Here's how the part is built. I have some questions about the finished solid (model axes, mm). Face numbers are marked on the shaded views. Give positions to 0.01 mm unless a question says otherwise; leave off trailing zeros. Loops run counter-clockwise (first coordinate to the right, second up) from the corner with the lowest first, then second, coordinate; pieces in that order, holes last. Notation, with made-up numbers: (75, -10.75) - (122, -10.75) arc R26 cw to (122, 13.25) - close; hole circle Ø9 at (-3, 63). An arc over 180 degrees is marked (long way). Use one line per item in the form item = value.
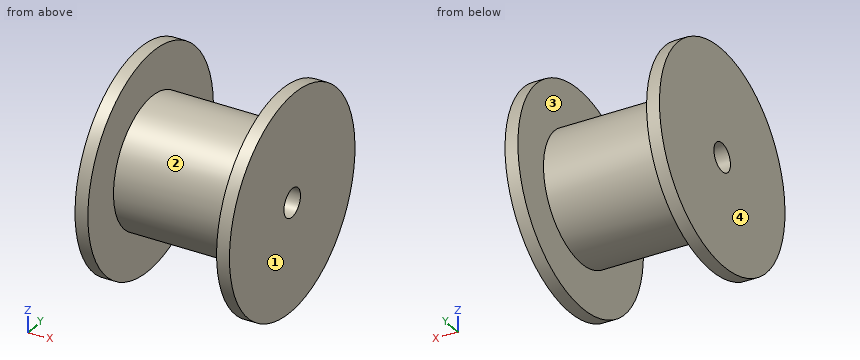
from build123d import *

# Parameters (mm, degrees)
CROQUIS1_R              = 76
SALIENTE_EXTRUIR1_DEPTH = 9
CROQUIS2_R              = 45
SALIENTE_EXTRUIR2_DEPTH = 90
CROQUIS3_R              = 76
SALIENTE_EXTRUIR3_DEPTH = 9
CROQUIS4_R              = 10
CORTAR_EXTRUIR1_DEPTH   = 108


with BuildPart() as part:
    # Croquis1 → Saliente-Extruir1 (new body)
    with BuildSketch(Plane(origin=(0, 0, 0), x_dir=(0, 0, -1), z_dir=(1, 0, 0))):
        Circle(CROQUIS1_R)
    extrude(amount=SALIENTE_EXTRUIR1_DEPTH)

    # Croquis2 → Saliente-Extruir2 (add)
    with BuildSketch(Plane(origin=(9, 0, 0), x_dir=(0, 0, -1), z_dir=(1, 0, 0))):
        with Locations(Location((0, 0, 0), (0, 0, 180))):
            Circle(CROQUIS2_R)
    extrude(amount=SALIENTE_EXTRUIR2_DEPTH)

    # Croquis3 → Saliente-Extruir3 (add)
    with BuildSketch(Plane(origin=(99, 0, 0), x_dir=(0, 0, -1), z_dir=(1, 0, 0))):
        Circle(CROQUIS3_R)
    extrude(amount=SALIENTE_EXTRUIR3_DEPTH)

    # Croquis4 → Cortar-Extruir1 (cut)
    with BuildSketch(Plane(origin=(108, 0, 0), x_dir=(0, 0, -1), z_dir=(1, 0, 0))):
        Circle(CROQUIS4_R)
    extrude(amount=-CORTAR_EXTRUIR1_DEPTH, mode=Mode.SUBTRACT)


solid = part.part
(1) If I drill on probe 1 along X at (y, z) = (12.5, 46.5); probe 2 along Y at (x, z) = (70.5, 0); probe 3 along Y at (x, z) = (22, -5), over which ranges is the centre line in solid material (lowest first)?
Geometry says:
probe_1 = 0 to 9, 99 to 108
probe_2 = -45 to -10, 10 to 45
probe_3 = -44.72 to -8.66, 8.66 to 44.72
(2) If we section it at C-C (x = 16.5): List the corners of the cut face in (y, z) for me, plus the area to 3 significant figures.
Geometry says:
outline = circle Ø90 at (0, 0); hole circle Ø20 at (0, 0)
area = 6,050 mm²
(3) For P1, Ø4, axis at x = 38, y = -29, coming from the +Z side; P2, Ø8, axis at x = 68.5, z = 18, coming from the -Y side; P3, Ø1.5, axis at x = 22.5, z = 21, coming from the +Y side, each with a flat end and sliding along its axis, tell me the tip position at first contact or that it passes through.
Geometry says:
P1 = 36
P2 = -42.77
P3 = 40.19
(4) If we section it at A-A (z = 0): List the corners of the cut face in (x, y) for me.
Geometry says:
outline = (0, -76) - (9, -76) - (9, -45) - (99, -45) - (99, -76) - (108, -76) - (108, -10) - (0, -10) - close; (0, 10) - (108, 10) - (108, 76) - (99, 76) - (99, 45) - (9, 45) - (9, 76) - (0, 76) - close
(5) If we section it at D-D (z = 59): List the corners of the cut face in (x, y) for me.
Geometry says:
outline = (0, -47.91) - (9, -47.91) - (9, 47.91) - (0, 47.91) - close; (99, -47.91) - (108, -47.91) - (108, 47.91) - (99, 47.91) - close
(6) Thinking about a two-plate mould opening in X: for the marked faces 1, 2, 3 and 4, which applies, pulls with the +X half, pulls with the -X half, needs draft (parallel to the pull), parting line crosses it, or undercut?
Geometry says:
face_1 = pulls with the +X half
face_2 = undercut
face_3 = undercut
face_4 = pulls with the -X half
